```python
from build123d import *

# Parameters (mm, degrees)
SKETCH1_R           = 11.2
BOSS_EXTRUDE1_DEPTH = 50.8


with BuildPart() as part:
    # Sketch1 → Boss-Extrude1 (new body)
    with BuildSketch(Plane.XY):
        with BuildLine():
            Line((-25.4, -19.455), (-25.4, 19.455))
            Line((-25.4, 19.455), (-25.4, 39.031999962))
            ThreePointArc((-25.4, 39.031999962), (-24.507261469, 41.187261431), (-22.352, 42.079999962))
            Line((-22.352, 42.079999962), (16.407, 42.079999962))
            ThreePointArc((16.407, 42.079999962), (18.562261469, 41.187261431), (19.455, 39.031999962))
            Line((19.455, 39.031999962), (19.455, 19.455))
            Line((19.455, 19.455), (19.455, 0))
            Line((19.455, 0), (19.455, -13.74))
            ThreePointArc((19.455, -13.74), (17.781115254, -17.781115254), (13.74, -19.455))
            Line((13.74, -19.455), (0, -19.455))
            Line((0, -19.455), (-16.002, -19.455))
            ThreePointArc((-16.002, -19.455), (-18.157261469, -20.347738531), (-19.05, -22.503))
            Line((-19.05, -22.503), (-19.05, -70.781999962))
            ThreePointArc((-19.05, -70.781999962), (-19.942738531, -72.937261431), (-22.098, -73.829999962))
            Line((-22.098, -73.829999962), (-22.352, -73.829999962))
            ThreePointArc((-22.352, -73.829999962), (-24.507261469, -72.937261431), (-25.4, -70.781999962))
            Line((-25.4, -70.781999962), (-25.4, -19.455))
        make_face()
        Circle(SKETCH1_R, mode=Mode.SUBTRACT)
    extrude(amount=BOSS_EXTRUDE1_DEPTH)


solid = part.part
```
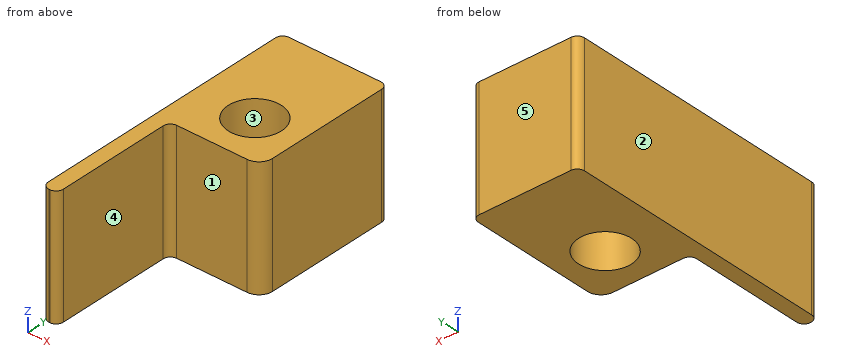
CAD build for the part. Positions are in the model's coordinates, mm. Face numbers are marked on the shaded views. A direction names the side the tool comes from. Round coordinates to 2 decimals unless told otherwise and drop trailing zeros. Order: outer loops, then holes, each group sorted by start corner. A loop starts at its lowest first (then second) coordinate and runs counter-clockwise, first axis right, second up.
Item 1: Saw through at A-A on y = 0. Write the cut outline in (x, z) (3 decimals).
Item 2: Saw through at C-C on z = 15.5. Write the cut outline in (x, y) (3 decimals).
Item 3: Pin check, flat tips, straight feed: pin 1 (4 mm diameter, centred on x = 6, y = 12, fed in from -Z); pin 2 (6 mm diameter, centred on x = -15.5, z = 15, fed in from -Y); pin 3 (10 mm diameter, centred on x = 5.5, z = 17.5, fed in from -Y) (3 decimals); pin 4 (10 mm diameter, centred on y = -47.5, z = 35, fed in from +X). Stop position of each tip, or through.
Item 4: Saw through at D-D on y = -61. Write the cut outline in (x, z), then the cut area to 3 significant figures.
Item 5: Probe line 1 along Y through (x, z) = (0, 31) (3 decimals); line 2 along Y through (x, z) = (13, 17) (3 decimals); line 3 along X through (y, z) = (-42.5, 25.5). List the from-to ranges inside material, lowest first.
Item 6: Tool access for the marked faces 4 and 5: list every direction of +Z, -Z, +X, -X, +Y, -Y with a clear straight run to the whole face (end or side of a thin tool).
Item 7: Mould opens along X. For the marked faces 1, 2 and 3 say: pulls with the +X half, pulls with the -X half, needs draft (parallel to the pull), parting line crosses it, or undercut.
Item 8: Saw through at B-B on x = 0. Write the cut outline in (y, z) (3 decimals).
Reported:
1. outline: (-25.4, 0) - (-11.2, 0) - (-11.2, 50.8) - (-25.4, 50.8) - close; (11.2, 0) - (19.455, 0) - (19.455, 50.8) - (11.2, 50.8) - close
2. outline: (-25.4, -70.782) arc R3.048 ccw to (-22.352, -73.83) - (-22.098, -73.83) arc R3.048 ccw to (-19.05, -70.782) - (-19.05, -22.503) arc R3.048 cw to (-16.002, -19.455) - (13.74, -19.455) arc R5.715 ccw to (19.455, -13.74) - (19.455, 39.032) arc R3.048 ccw to (16.407, 42.08) - (-22.352, 42.08) arc R3.048 ccw to (-25.4, 39.032) - close; hole circle Ø22.4 at (0, 0)
3. pin 1: stops at z = 0
3. pin 2: stops at y = -20.76
3. pin 3: stops at y = -19.455
3. pin 4: stops at x = -19.05
4. outline: (-25.4, 0) - (-19.05, 0) - (-19.05, 50.8) - (-25.4, 50.8) - close
4. area: 323 mm2
5. line 1: y = -19.455 to -11.2, 11.2 to 42.08
5. line 2: y = -19.455 to 42.08
5. line 3: x = -25.4 to -19.05
6. face 4: +Z, -Z, +X, -Y
6. face 5: +Z, -Z, +X, -X, +Y
7. face 1: needs draft
7. face 2: pulls with the -X half
7. face 3: undercut
8. outline: (-19.455, 0) - (-11.2, 0) - (-11.2, 50.8) - (-19.455, 50.8) - close; (11.2, 0) - (42.08, 0) - (42.08, 50.8) - (11.2, 50.8) - close
